Autodesk Inventor part; units mm, degrees
ref_plane "Work Plane1" through (31.5, 0, 0) normal (1, 0, 0) x (0, 0, -1)
ref_plane "Work Plane2" through (-33.5, 0, -33.5) normal (0, 0, 1) x (1, 0, 0)
ref_plane "YZ Plane" through (0, 0, 0) normal (1, 0, 0) x (0, 1, 0)
sketch "Sketch1" plane through (0, 0, 0) normal (1, 0, 0) x (0, 1, 0)
  line L0 (-2.6, 0) -> (15.6, 0)
  line L1 (0, -98.5723) -> (0, 16.4287)
  line L2 (13, 0) -> (0, 0)
  line L3 (13, 0) -> (13, -80)
  line L4 (0, 0) -> (0, -67)
  line L5 (0, -67) -> (6.5, -73.5)
  line L6 (0, -67) -> (9.1924, -67) construction
  arc A0 (6.5, -73.5) -> (13, -80) centre (11.1419, -75.3581) ccw
  circle A1 centre (9.75, -77.5) radius 1.625
  dimension "d2" = 13
  dimension "d6" = 80
  dimension "d7" = 67
  dimension "d8" = 45
  dimension "d9" = 6.5
  dimension "d10" = 5
  dimension "d11" = 3.25
  dimension "d12" = 3.25
  dimension "d13" = 2.5
extrude "Extrusion1" add sketch "Sketch1" along normal mid plane 67
sketch "Sketch3" plane through (-33.5, 13, 0) normal (0, 1, 0) x (1, 0, 0)
  line L0 (0, 73.5) -> (67, 73.5)
  line L1 (0, 0) -> (0, 80)
  line L2 (67, 80) -> (67, 0)
  line L3 (1.5, 73.5) -> (0, 73.5)
  line L4 (0, 73.5) -> (0, 80.5)
  line L5 (0, 80.5) -> (1.5, 80.5)
  line L6 (1.5, 80.5) -> (1.5, 73.5)
  line L7 (7.5, 73.5) -> (3.5, 73.5)
  line L8 (3.5, 73.5) -> (3.5, 80.5)
  line L9 (3.5, 80.5) -> (7.5, 80.5)
  line L10 (7.5, 80.5) -> (7.5, 73.5)
  line L11 (19.5, 73.5) -> (9.5, 73.5)
  line L12 (9.5, 73.5) -> (9.5, 80.5)
  line L13 (9.5, 80.5) -> (19.5, 80.5)
  line L14 (19.5, 80.5) -> (19.5, 73.5)
  line L15 (25.5, 80.5) -> (21.5, 80.5)
  line L16 (21.5, 80.5) -> (21.5, 73.5)
  line L17 (21.5, 73.5) -> (25.5, 73.5)
  line L18 (25.5, 73.5) -> (25.5, 80.5)
  line L19 (37.5, 73.5) -> (27.5, 73.5)
  line L20 (27.5, 73.5) -> (27.5, 80.5)
  line L21 (27.5, 80.5) -> (37.5, 80.5)
  line L22 (37.5, 80.5) -> (37.5, 73.5)
  line L23 (43.5, 73.5) -> (39.5, 73.5)
  line L24 (39.5, 73.5) -> (39.5, 80.5)
  line L25 (39.5, 80.5) -> (43.5, 80.5)
  line L26 (43.5, 80.5) -> (43.5, 73.5)
  line L27 (55.5, 73.5) -> (45.5, 73.5)
  line L28 (45.5, 73.5) -> (45.5, 80.5)
  line L29 (45.5, 80.5) -> (55.5, 80.5)
  line L30 (55.5, 80.5) -> (55.5, 73.5)
  line L31 (61.5, 73.5) -> (57.5, 73.5)
  line L32 (57.5, 73.5) -> (57.5, 80.5)
  line L33 (57.5, 80.5) -> (61.5, 80.5)
  line L34 (61.5, 80.5) -> (61.5, 73.5)
  line L35 (67, 73.5) -> (63.5, 73.5)
  line L36 (63.5, 73.5) -> (63.5, 80.5)
  line L37 (63.5, 80.5) -> (67, 80.5)
  line L38 (67, 80.5) -> (67, 73.5)
  point P0 (33.5, 0)
  dimension "d52" = 1.5
  dimension "d53" = 7
  dimension "d54" = 4
  dimension "d55" = 7
  dimension "d56" = 2
  dimension "d57" = 10
  dimension "d58" = 7
  dimension "d59" = 2
  dimension "d60" = 4
  dimension "d61" = 7
  dimension "d62" = 2
  dimension "d63" = 10
  dimension "d64" = 7
  dimension "d65" = 2
  dimension "d66" = 4
  dimension "d67" = 2
  dimension "d68" = 7
  dimension "d69" = 10
  dimension "d70" = 7
  dimension "d71" = 2
  dimension "d72" = 4
  dimension "d73" = 7
  dimension "d74" = 2
  dimension "d75" = 7
  dimension "d76" = 2
extrude "Extrusion3" cut sketch "Sketch3" against normal blind 13
ref_plane "Work Plane1" through (31.5, 0, 0) normal (1, 0, 0) x (0, 0, -1)
sketch "Sketch4" plane through (31.5, 0, 0) normal (1, 0, 0) x (0, 0, -1)
  line L0 (2, 13) -> (2, 2)
  line L1 (2, 2) -> (66.1716, 2)
  line L2 (0, 13) -> (73.5, 13)
  line L3 (0, 0) -> (0, 13)
  line L4 (67, 0) -> (0, 0)
  line L5 (73.5, 6.5) -> (67, 0)
  line L6 (71.5, 7.3284) -> (71.5, 13)
  line L7 (73.5, 13) -> (73.5, 6.5)
  line L8 (71.5, 7.3284) -> (66.1716, 2)
  dimension "d80" = 2
  dimension "d81" = 2
  dimension "d82" = 2
  dimension "d83" = 2
  dimension "d84" = 2
extrude "Extrusion4" cut sketch "Sketch4" against normal blind 63 contours L2 L6 L8 L1 L0
sketch "Sketch5" plane through (4, 13, -73.5) normal (0, 0, -1) x (-1, 0, 0)
  line L0 (4, -15.6) -> (4, 2.6)
  line L1 (50.9, -13) -> (-42.9, -13)
  line L2 (-29.5, -6.5) -> (-29.5, 0)
  line L3 (37.5, 0) -> (37.5, -6.5)
  line L4 (-18, 0) -> (-8, 0)
  circle A0 centre (-23, -3) radius 0.75
  circle A1 centre (-5, -3) radius 0.75
  circle A2 centre (13, -3) radius 0.75
  line L5 (0, 0) -> (10, 0)
  circle A3 centre (31, -3) radius 0.75
  dimension "d88" = 1.5
  dimension "d89" = 3
  dimension "d90" = 6.5
  dimension "d94" = 1.5
  dimension "d95" = 3
  dimension "d96" = 18
  dimension "d100" = 1.5
  dimension "d101" = 3
  dimension "d102" = 18
  dimension "d106" = 1.5
  dimension "d108" = 3
  dimension "d109" = 18
ref_plane "Work Plane2" through (-33.5, 0, -33.5) normal (0, 0, 1) x (1, 0, 0)
extrude "Extrusion11" cut sketch "Sketch5" against normal blind 2
sketch "Sketch13" plane through (22, 13, -73.5) normal (0, 0, -1) x (-1, 0, 0)
  line L0 (55.5, -13) -> (-11.5, -13)
  circle A0 centre (-5, -10) radius 0.75
  circle A1 centre (13, -10) radius 0.75
  circle A2 centre (31, -10) radius 0.75
  circle A3 centre (49, -10) radius 0.75
  line L1 (-11.5, -13) -> (-11.5, -6.5)
  line L2 (55.5, -6.5) -> (55.5, -13)
  point P0 (22, -13)
  dimension "d159" = 1.5
  dimension "d160" = 1.5
  dimension "d161" = 1.5
  dimension "d162" = 1.5
  dimension "d163" = 3
  dimension "d164" = 6.5
  dimension "d165" = 3
  dimension "d166" = 18
  dimension "d167" = 3
  dimension "d168" = 18
  dimension "d169" = 3
  dimension "d170" = 18
extrude "Extrusion12" cut sketch "Sketch13" against normal through all
sketch "Sketch22" plane through (-33.5, 13, 0) normal (0, 1, 0) x (1, 0, 0)
  line L0 (65, 2) -> (2, 2)
  line L1 (2, 9) -> (11, 9)
  line L2 (11, 9) -> (11, 2)
  line L3 (11, 2) -> (2, 2)
  line L4 (2, 2) -> (2, 9)
  circle A0 centre (6.5, 67.1716) radius 0.75
  line L5 (65, 2) -> (65, 66.1716)
  line L6 (65, 66.1716) -> (2, 66.1716)
  line L7 (2, 66.1716) -> (2, 2)
  line L8 (65, 2) -> (2, 2)
  line L9 (20, 9) -> (29, 9)
  line L10 (29, 9) -> (29, 2)
  line L11 (29, 2) -> (20, 2)
  line L12 (20, 2) -> (20, 9)
  line L13 (56, 9) -> (65, 9)
  line L14 (65, 9) -> (65, 2)
  line L15 (65, 2) -> (56, 2)
  line L16 (56, 2) -> (56, 9)
  line L17 (38, 9) -> (47, 9)
  line L18 (47, 9) -> (47, 2)
  line L19 (47, 2) -> (38, 2)
  line L20 (38, 2) -> (38, 9)
  dimension "d275" = 9
  dimension "d278" = 7
  dimension "d279" = 9
  dimension "d280" = 7
  dimension "d281" = 9
  dimension "d282" = 9
  dimension "d283" = 7
  dimension "d284" = 9
  dimension "d285" = 7
  dimension "d286" = 9
extrude "Extrusion19" add sketch "Sketch22" against normal blind 7 contours L0 L16 L13 L5 | L0 L20 L17 L18 | L0 L12 L9 L10 | L1 L2 L0 L4
sketch "Sketch23" plane through (31.5, 0, 0) normal (-1, 0, 0) x (0, 0, 1)
  line L0 (-9.5, 11) -> (-2, 11)
  line L1 (-2, 11) -> (-2, 8)
  line L2 (-2, 8) -> (-9.5, 8)
  line L3 (-9.5, 8) -> (-9.5, 11)
  line L4 (-2, 13) -> (-2, 6)
  line L5 (-2, 13) -> (-9, 13)
  point P0 (0, 0)
  dimension "d289" = 7.5
  dimension "d290" = 3
  dimension "d291" = 2
extrude "Extrusion20" cut sketch "Sketch23" along normal blind 63
sketch "Sketch24" plane through (-33.5, 13, 0) normal (0, 1, 0) x (1, 0, 0)
  line L0 (56, 9) -> (65, 9)
  line L1 (56, 2) -> (56, 9)
  line L2 (47, 9) -> (47, 2)
  line L3 (38, 9) -> (47, 9)
  line L4 (29, 9) -> (29, 2)
  line L5 (20, 9) -> (29, 9)
  line L6 (11, 9) -> (11, 2)
  line L7 (2, 9) -> (11, 9)
  circle A0 centre (60.5, 5.5) radius 1.625
  circle A1 centre (42.5, 5.5) radius 1.625
  circle A2 centre (24.5, 5.5) radius 1.625
  circle A3 centre (6.5, 5.5) radius 1.625
  point P0 (33.5, 0)
  dimension "d294" = 3.25
  dimension "d295" = 3.5
  dimension "d296" = 4.5
  dimension "d297" = 3.25
  dimension "d298" = 3.5
  dimension "d299" = 4.5
  dimension "d301" = 3.25
  dimension "d302" = 3.5
  dimension "d303" = 4.5
  dimension "d304" = 3.25
  dimension "d305" = 3.5
  dimension "d306" = 4.5
extrude "Extrusion21" cut sketch "Sketch24" against normal blind 7
sketch "Sketch26" plane through (31.5, 2, -2) normal (0, 0, -1) x (-1, 0, 0)
  line L0 (9, 6) -> (9, 4)
  line L1 (9, 11) -> (9, 9)
  line L2 (0, 6) -> (9, 6)
  line L3 (0, 9) -> (9, 9)
  line L4 (0, 9) -> (9, 9)
  line L5 (18, 9) -> (18, 11)
  line L6 (18, 6) -> (27, 6)
  line L7 (36, 6) -> (45, 6)
  line L8 (54, 6) -> (63, 6)
  circle A0 centre (13.5, 6) radius 1.625
  circle A1 centre (31.5, 6) radius 1.625
  circle A2 centre (49.5, 6) radius 1.625
  point P0 (31.5, -2)
  dimension "d311" = 3.25
  dimension "d313" = 4.5
  dimension "d314" = 3.25
  dimension "d316" = 4.5
  dimension "d317" = 3.25
  dimension "d319" = 4.5
extrude "Extrusion22" cut sketch "Sketch26" against normal blind 2
properties part number "palm"
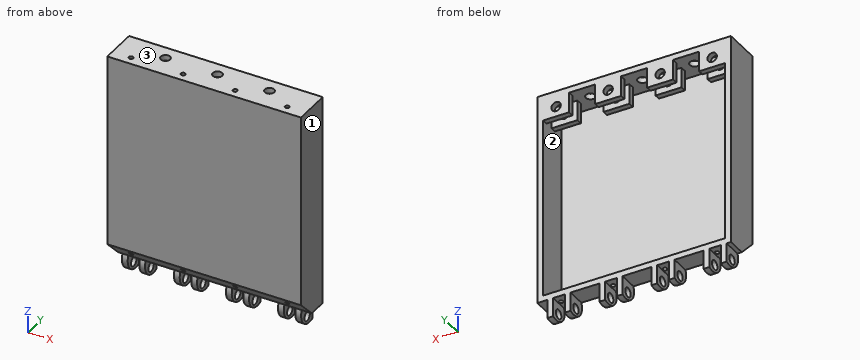
Geometry check sheet. Reference: the model listing, model coordinates, mm. Face numbers are marked on the shaded views. Give positions to 0.01 mm unless a question says otherwise; leave off trailing zeros. Order: outer loops, then holes, each group sorted by start corner. A loop starts at its lowest first (then second) coordinate and runs counter-clockwise, first axis right, second up. Notation, with made-up numbers: M -26,26 L -5,26 A17 cw -5,37 Z; hole C 86.25,-7.75 d6. An arc over 180 degrees is marked long. Use a Markdown table: item, result.
Item 1: Section check A-A (x = -18). Record the cut outline in (y, z) (3 decimals).
Answers follow:
| item | result |
|---|---|
| outline | M 0,-67 L 6.5,-73.5 L 13,-73.5 L 13,-71.5 L 7.328,-71.5 L 2,-66.172 L 2,-2 L 6.375,-2 L 6.375,0 L 0,0 Z; M 9.625,-2 L 13,-2 L 13,0 L 9.625,0 Z |
Item 2: Section check B-B (z = -27.5). Record the cut outline in (x, y).
Answers follow:
| item | result |
|---|---|
| outline | M -33.5,0 L 33.5,0 L 33.5,13 L 31.5,13 L 31.5,2 L -31.5,2 L -31.5,13 L -33.5,13 Z |
Item 3: Depth check by flat-ended pin: P1, Ø2, axis at y = 8, z = -75, coming from the -X side; P2, Ø3.5, axis at y = 9.75, z = -77.5, coming from the +X side; P3, Ø1, axis at x = 2, z = -25, coming from the +Y side; P4, Ø0.9, axis at x = -27, y = 3, coming from the -Z side. Enter the tip coordinate at first touch or a pass-through.
Answers follow:
| item | result |
|---|---|
| P1 | stops at x = -32 |
| P2 | stops at x = 30 |
| P3 | stops at y = 2 |
| P4 | passes through |
Item 4: Draft check along Z on the marked faces 1, 2 and 3. Enter one of: +Z half, -Z half, draft (parallel to the pull), parting line (faces both ways), or undercut.
Answers follow:
| item | result |
|---|---|
| face 1 | draft |
| face 2 | undercut |
| face 3 | +Z half |
Item 5: Material ranges on line 1 along X through (y, z) = (3, -68.75); line 2 along Z through (x, y) = (27, 11.4) (3 decimals); line 3 along X through (y, z) = (4.5, -33.5), recorded low to high.
Answers follow:
| item | result |
|---|---|
| line 1 | x = -33.5 to -27.75, -26.25 to -9.75, -8.25 to 8.25, 9.75 to 26.25, 27.75 to 33.5 |
| line 2 | z = -73.5 to -71.5, -9 to -7.125, -3.875 to 0 |
| line 3 | x = -33.5 to -31.5, 31.5 to 33.5 |
